Geometry check sheet. Reference: the model listing, model coordinates, mm. A direction names the side the tool comes from. Give positions to 0.01 mm unless a question says otherwise; leave off trailing zeros. Write each loop counter-clockwise with the first axis right and the second up, starting at its lowest first coordinate (ties: lowest second). Pieces come first, ordered by that corner, then holes. Notation, with made-up numbers: (-25.5, -18.5) - (13.5, -18.5) arc R22 cw to (13.5, 3.5) - close; hole circle Ø9 at (87.25, 20.25). An arc over 180 degrees is marked (long way). Write item = value, one per line. Start each with the question number.
(1) Thickness scan on L1, parallel to Z at x = -9.75, y = -16.25; L2, parallel to X at y = -1.05, z = -6; L3, parallel to Y at x = -10, z = 6. Record the ranges inside material, lowest first.
(2) Draft check along Y on faces 4 (the cylindrical face through (-10.27, -0.74, -7.55)), 5 (the flat face through (3, 0, -4)), 6 (the cylindrical face through (7.179, -6.934, -21.16)), 7 (the cylindrical face through (-7.27, -6.9, -21.16)). Enter one of: pulls with the +Y half, pulls with the -Y half, needs draft (parallel to the pull), parting line crosses it, or undercut.
(3) Section check C-C, the plane z = 7. Enter the section's corners in (x, y), plus the area to 3 significant figures.
(4) Access from +Z, -Z, +X, -X, +Y, -Y to the whole of each face (thin tool, end or side, straight path). Record for faces 1 (the cylindrical face through (0.141, -1.996, 19.929)), 2 (the flat face through (10.1, -8, 21)), 3 (the cylindrical face through (-0.59, -7.67, 21.14)).
(5) Section check D-D, the plane x = -2.25. Enter the section's corners in (y, z), plus the area to 3 significant figures.
(6) Depth check by flat-ended pin: pin 1 Ø10.5 at (y, z) = (-6.5, 18.5) entering from -X; pin 2 Ø1.3 at (x, y) = (0, -8.6) entering from +Z; pin 3 Ø12 at (x, z) = (-7.5, -6) entering from -Y; pin 4 Ø2.5 at (x, z) = (-6, -6) entering from -Y. Enter the tip coordinate at first touch or a pass-through.
(7) Section check B-B, the plane y = -12.5. Enter the section's corners in (x, z), plus the area to 3 significant figures.
(8) Section check A-A, the plane y = -23.05. Enter the section's corners in (x, z), plus the area to 3 significant figures.
```python
from build123d import *

# Parameters (mm, degrees)
SKETCH1_W                      = 20.2
SKETCH1_H                      = 40.8
BASE_FLANGE1_DEPTH             = 1.5
EDGE_FLANGE1_STRIP_W           = 9.3
EDGE_FLANGE1_STRIP_H           = 1.5
EDGE_FLANGE1_STRIP_CUT_DEPTH   = 20.2
EDGE_FLANGE1_STRIP_2_W         = 9.3
EDGE_FLANGE1_STRIP_2_H         = 1.5
EDGE_FLANGE1_STRIP_CUT_2_DEPTH = 20.2
EDGE_FLANGE1_DEPTH             = 20.2
EDGE_FLANGE1_BEND_DEPTH        = 20.2
CUT_EXTRUDE1_REACH             = 53.952
SKETCH12_R                     = 1.1
FILLET1_R                      = 2
F_2_0MM_DOWEL_HOLE1_D          = 2.2
F_2_0MM_DOWEL_HOLE1_DEPTH      = 1.5
SKETCH15_R                     = 12.5
TAB1_DEPTH                     = 1.5
FILLET2_R                      = 5
CUT_EXTRUDE2_REACH             = 38.256
SKETCH18_R                     = 1.6
SKETCH18_R_2                   = 4.75


# Sheet-metal steps are written as plain solids
with BuildPart() as part:
    # Sketch1 → Base-Flange1 (new body)
    with BuildSketch(Plane(origin=(0, 0, 0), x_dir=(1, 0, 0), z_dir=(0, 1, 0))):
        Rectangle(SKETCH1_W, SKETCH1_H)
    extrude(amount=-BASE_FLANGE1_DEPTH)

    # Edge-Flange1 strip (across the edge) → Edge-Flange1 strip cut (cut)
    with BuildSketch(Plane(origin=(10.1, -1.5, 20.4), x_dir=(0, 0, -1), z_dir=(-1, 0, 0))):
        with Locations((-3, -0.75)):
            Rectangle(EDGE_FLANGE1_STRIP_W, EDGE_FLANGE1_STRIP_H)
    extrude(amount=EDGE_FLANGE1_STRIP_CUT_DEPTH, mode=Mode.SUBTRACT)

    # Edge-Flange1 strip 2 (across the edge) → Edge-Flange1 strip cut 2 (cut)
    with BuildSketch(Plane(origin=(-10.1, -1.5, -20.4), x_dir=(0, 0, 1), z_dir=(1, 0, 0))):
        with Locations((-3, -0.75)):
            Rectangle(EDGE_FLANGE1_STRIP_2_W, EDGE_FLANGE1_STRIP_2_H)
    extrude(amount=EDGE_FLANGE1_STRIP_CUT_2_DEPTH, mode=Mode.SUBTRACT)

    # Edge-Flange1 section (across the edge) → Edge-Flange1 (add)
    with BuildSketch(Plane(origin=(10.1, -1.5, 20.4), x_dir=(0, 0, -1), z_dir=(-1, 0, 0))):
        with BuildLine():
            Line((-1.5, 1.65), (-1.5, 24.55))
            Line((-1.5, 24.55), (0, 24.55))
            Line((0, 24.55), (0, 1.65))
            ThreePointArc((0, 1.65), (0.483273811, 0.483273811), (1.65, 0))
            Line((1.65, 0), (1.65, -1.5))
            ThreePointArc((1.65, -1.5), (-0.577386361, -0.577386361), (-1.5, 1.65))
        make_face()
    extrude(amount=EDGE_FLANGE1_DEPTH)

    # Edge-Flange1 section 2 (across the edge) → Edge-Flange1 bend (add)
    with BuildSketch(Plane(origin=(-10.1, -1.5, -20.4), x_dir=(0, 0, 1), z_dir=(1, 0, 0))):
        with BuildLine():
            Line((-1.5, 1.65), (-1.5, 24.55))
            Line((-1.5, 24.55), (0, 24.55))
            Line((0, 24.55), (0, 1.65))
            ThreePointArc((0, 1.65), (0.483273811, 0.483273811), (1.65, 0))
            Line((1.65, 0), (1.65, -1.5))
            ThreePointArc((1.65, -1.5), (-0.577386361, -0.577386361), (-1.5, 1.65))
        make_face()
    extrude(amount=EDGE_FLANGE1_BEND_DEPTH)

    # Sketch12 → Cut-Extrude1 (cut, up to next)
    with BuildSketch(Plane(origin=(0, 0, -21.9), x_dir=(-1, 0, 0), z_dir=(0, 0, -1)), mode=Mode.PRIVATE) as cut_extrude1_sk1:
        with Locations(Location((-7.6, -7.95, 0), (0, 0, 90))):
            Circle(SKETCH12_R)
    cut_extrude1_tool1 = extrude(cut_extrude1_sk1.sketch, amount=-CUT_EXTRUDE1_REACH, mode=Mode.PRIVATE) & part.part
    # Sketch12 → Cut-Extrude1 (cut, up to next)
    with BuildSketch(Plane(origin=(0, 0, -21.9), x_dir=(-1, 0, 0), z_dir=(0, 0, -1)), mode=Mode.PRIVATE) as cut_extrude1_sk2:
        with Locations(Location((7.6, -7.95, 0), (0, 0, 90))):
            Circle(SKETCH12_R)
    cut_extrude1_tool2 = extrude(cut_extrude1_sk2.sketch, amount=-CUT_EXTRUDE1_REACH, mode=Mode.PRIVATE) & part.part
    # Sketch12 → Cut-Extrude1 (cut, up to next)
    with BuildSketch(Plane(origin=(0, 0, -21.9), x_dir=(-1, 0, 0), z_dir=(0, 0, -1)), mode=Mode.PRIVATE) as cut_extrude1_sk3:
        with Locations(Location((7.6, -23.05, 0), (0, 0, 90))):
            Circle(SKETCH12_R)
    cut_extrude1_tool3 = extrude(cut_extrude1_sk3.sketch, amount=-CUT_EXTRUDE1_REACH, mode=Mode.PRIVATE) & part.part
    # Sketch12 → Cut-Extrude1 (cut, up to next)
    with BuildSketch(Plane(origin=(0, 0, -21.9), x_dir=(-1, 0, 0), z_dir=(0, 0, -1)), mode=Mode.PRIVATE) as cut_extrude1_sk4:
        with Locations(Location((-7.6, -23.05, 0), (0, 0, 90))):
            Circle(SKETCH12_R)
    cut_extrude1_tool4 = extrude(cut_extrude1_sk4.sketch, amount=-CUT_EXTRUDE1_REACH, mode=Mode.PRIVATE) & part.part
    add(cut_extrude1_tool1.solids().sort_by_distance((7.6, -7.95, -21.9))[0], mode=Mode.SUBTRACT)
    add(cut_extrude1_tool2.solids().sort_by_distance((-7.6, -7.95, -21.9))[0], mode=Mode.SUBTRACT)
    add(cut_extrude1_tool3.solids().sort_by_distance((-7.6, -23.05, -21.9))[0], mode=Mode.SUBTRACT)
    add(cut_extrude1_tool4.solids().sort_by_distance((7.6, -23.05, -21.9))[0], mode=Mode.SUBTRACT)

    # Fillet1
    fillet1_edges = [part.edges().sort_by_distance(p)[0] for p in [
        (10.1, -26.05, 21.15),
        (-10.1, -26.05, 21.15),
        (-10.1, -26.05, -21.15),
        (10.1, -26.05, -21.15),
    ]]
    fillet(fillet1_edges, radius=FILLET1_R)

    # Ø2.0mm Dowel Hole1
    with Locations(Plane.XY.offset(21.9)):
        with Locations((-7, -15.6), (0, -8.6), (7, -15.6)):
            Hole(F_2_0MM_DOWEL_HOLE1_D / 2, depth=F_2_0MM_DOWEL_HOLE1_DEPTH)

    # Sketch15 → Tab1 (add)
    with BuildSketch(Plane(origin=(0, 0, 0), x_dir=(1, 0, 0), z_dir=(0, 1, 0))):
        Circle(SKETCH15_R)
    extrude(amount=-TAB1_DEPTH)

    # Fillet2
    fillet2_edges = [part.edges().sort_by_distance(p)[0] for p in [
        (-10.1, -0.75, -7.364781056),
        (-10.1, -0.75, 7.364781056),
        (10.1, -0.75, -7.364781056),
        (10.1, -0.75, 7.364781056),
    ]]
    fillet(fillet2_edges, radius=FILLET2_R)

    # Sketch18 → Cut-Extrude2 (cut, up to next)
    with BuildSketch(Plane(origin=(0, 0, 0), x_dir=(1, 0, 0), z_dir=(0, 1, 0)), mode=Mode.PRIVATE) as cut_extrude2_sk1:
        with Locations(Location((-6, 6, 0), (0, 0, 270))):
            Circle(SKETCH18_R)
    cut_extrude2_tool1 = extrude(cut_extrude2_sk1.sketch, amount=-CUT_EXTRUDE2_REACH, mode=Mode.PRIVATE) & part.part
    # Sketch18 → Cut-Extrude2 (cut, up to next)
    with BuildSketch(Plane(origin=(0, 0, 0), x_dir=(1, 0, 0), z_dir=(0, 1, 0)), mode=Mode.PRIVATE) as cut_extrude2_sk2:
        with Locations(Location((6, 6, 0), (0, 0, 270))):
            Circle(SKETCH18_R)
    cut_extrude2_tool2 = extrude(cut_extrude2_sk2.sketch, amount=-CUT_EXTRUDE2_REACH, mode=Mode.PRIVATE) & part.part
    # Sketch18 → Cut-Extrude2 (cut, up to next)
    with BuildSketch(Plane(origin=(0, 0, 0), x_dir=(1, 0, 0), z_dir=(0, 1, 0)), mode=Mode.PRIVATE) as cut_extrude2_sk3:
        with Locations(Location((-6, -6, 0), (0, 0, 270))):
            Circle(SKETCH18_R)
    cut_extrude2_tool3 = extrude(cut_extrude2_sk3.sketch, amount=-CUT_EXTRUDE2_REACH, mode=Mode.PRIVATE) & part.part
    # Sketch18 → Cut-Extrude2 (cut, up to next)
    with BuildSketch(Plane(origin=(0, 0, 0), x_dir=(1, 0, 0), z_dir=(0, 1, 0)), mode=Mode.PRIVATE) as cut_extrude2_sk4:
        with Locations(Location((6, -6, 0), (0, 0, 270))):
            Circle(SKETCH18_R)
    cut_extrude2_tool4 = extrude(cut_extrude2_sk4.sketch, amount=-CUT_EXTRUDE2_REACH, mode=Mode.PRIVATE) & part.part
    # Sketch18 → Cut-Extrude2 (cut, up to next)
    with BuildSketch(Plane(origin=(0, 0, 0), x_dir=(1, 0, 0), z_dir=(0, 1, 0)), mode=Mode.PRIVATE) as cut_extrude2_sk5:
        with Locations(Location((0, 0, 0), (0, 0, 270))):
            Circle(SKETCH18_R_2)
    cut_extrude2_tool5 = extrude(cut_extrude2_sk5.sketch, amount=-CUT_EXTRUDE2_REACH, mode=Mode.PRIVATE) & part.part
    add(cut_extrude2_tool1.solids().sort_by_distance((-6, 0, -6))[0], mode=Mode.SUBTRACT)
    add(cut_extrude2_tool2.solids().sort_by_distance((6, 0, -6))[0], mode=Mode.SUBTRACT)
    add(cut_extrude2_tool3.solids().sort_by_distance((-6, 0, 6))[0], mode=Mode.SUBTRACT)
    add(cut_extrude2_tool4.solids().sort_by_distance((6, 0, 6))[0], mode=Mode.SUBTRACT)
    add(cut_extrude2_tool5.solids().sort_by_distance((0, 0, 0))[0], mode=Mode.SUBTRACT)


solid = part.part
```
Model answer:
q1.L1 = -21.9 to -20.4, 20.4 to 21.9
q1.L2 = -10.97 to -7.6, -4.4 to 4.4, 7.6 to 10.97
q1.L3 = -1.5 to 0
q2.face_4 = needs draft
q2.face_5 = pulls with the +Y half
q2.face_6 = undercut
q2.face_7 = undercut
q3.outline = (-10.45, -1.5) - (-7.25, -1.5) - (-7.25, 0) - (-10.45, 0) - close; (-4.75, -1.5) - (4.75, -1.5) - (4.75, 0) - (-4.75, 0) - close; (7.25, -1.5) - (10.45, -1.5) - (10.45, 0) - (7.25, 0) - close
q3.area = 23.9 mm²
q4.face_1 = +X, -X, -Y
q4.face_2 = +Z, +X, +Y, -Y
q4.face_3 = +Z
q5.outline = (-26.05, -21.9) - (-3.15, -21.9) arc R3.15 ccw to (0, -18.75) - (0, -4.18) - (-1.5, -4.18) - (-1.5, -18.75) arc R1.65 cw to (-3.15, -20.4) - (-26.05, -20.4) - close; (-26.05, 20.4) - (-3.15, 20.4) arc R1.65 cw to (-1.5, 18.75) - (-1.5, 4.18) - (0, 4.18) - (0, 18.75) arc R3.15 ccw to (-3.15, 21.9) - (-26.05, 21.9) - close
q5.area = 124 mm²
q6.pin_1 = -10.1
q6.pin_2 = -20.4
q6.pin_3 = -1.5
q6.pin_4 = through
q7.outline = (-10.1, -21.9) - (10.1, -21.9) - (10.1, -20.4) - (-10.1, -20.4) - close; (-10.1, 20.4) - (10.1, 20.4) - (10.1, 21.9) - (-10.1, 21.9) - close
q7.area = 60.6 mm²
q8.outline = (-10.1, -21.9) - (-8.7, -21.9) - (-8.7, -20.4) - (-10.1, -20.4) - close; (-10.1, 20.4) - (10.1, 20.4) - (10.1, 21.9) - (-10.1, 21.9) - close; (-6.5, -21.9) - (6.5, -21.9) - (6.5, -20.4) - (-6.5, -20.4) - close; (8.7, -21.9) - (10.1, -21.9) - (10.1, -20.4) - (8.7, -20.4) - close
q8.area = 54.0 mm²
